from build123d import *

# Parameters (mm, degrees)
BOX013_W               = 80
BOX013_H               = 4
BOX013_DEPTH           = 80
BOX013_PLACEMENT_ANGLE = 45
FILLET059_R            = 20
BOX017_W               = 80
BOX017_H               = 4
BOX017_DEPTH           = 80
BOX017_PLACEMENT_ANGLE = 45
FILLET060_R            = 20
BOX018_W               = 100
BOX018_H               = 4
BOX018_DEPTH           = 100
BOX018_PLACEMENT_ANGLE = 45
FILLET062_R            = 60
CYLINDER039_R          = 1.6
CYLINDER039_DEPTH      = 25
CYLINDER040_R          = 1.6
CYLINDER040_DEPTH      = 25
CYLINDER041_R          = 1.6
CYLINDER041_DEPTH      = 25
CYLINDER038_R          = 1.6
CYLINDER038_DEPTH      = 25
BOX014_W               = 100
BOX014_H               = 4
BOX014_DEPTH           = 100
BOX014_PLACEMENT_ANGLE = 45
FILLET061_R            = 60
BOX012_W               = 136
BOX012_H               = 4
BOX012_DEPTH           = 200
FILLET063_R            = 30
CHAMFER017_SIZE        = 2


with BuildPart() as fillet059:
    # Box013 → Box013 (new body)
    with BuildSketch(Plane.XY):
        with Locations((40, 2)):
            Rectangle(BOX013_W, BOX013_H)
    extrude(amount=BOX013_DEPTH)


with BuildPart() as fillet059_1:
    # Box013 placement: moved
    add(fillet059.part.moved(Location((-6.57, 0, 202))).rotate(Axis((-6.57, 0, 202), (0, 1, 0)), BOX013_PLACEMENT_ANGLE))

    # Fillet059
    fillet059_edges = [fillet059_1.edges().sort_by_distance(p)[0] for p in [
        (49.998542, 2, 145.431458),
    ]]
    fillet(fillet059_edges, radius=FILLET059_R)


with BuildPart() as fillet060:
    # Box017 → Box017 (new body)
    with BuildSketch(Plane.XY):
        with Locations((40, 2)):
            Rectangle(BOX017_W, BOX017_H)
    extrude(amount=BOX017_DEPTH)


with BuildPart() as fillet060_1:
    # Box017 placement: moved
    add(fillet060.part.moved(Location((-6.57, 0, -2))).rotate(Axis((-6.57, 0, -2), (0, 1, 0)), BOX017_PLACEMENT_ANGLE))

    # Fillet060
    fillet060_edges = [fillet060_1.edges().sort_by_distance(p)[0] for p in [
        (49.998542, 2, 54.568542),
    ]]
    fillet(fillet060_edges, radius=FILLET060_R)


with BuildPart() as fillet062:
    # Box018 → Box018 (new body)
    with BuildSketch(Plane.XY):
        with Locations((50, 2)):
            Rectangle(BOX018_W, BOX018_H)
    extrude(amount=BOX018_DEPTH)


with BuildPart() as fillet062_1:
    # Box018 placement: moved
    add(fillet062.part.moved(Location((48.67, 0, 100))).rotate(Axis((48.67, 0, 100), (0, 1, 0)), BOX018_PLACEMENT_ANGLE))

    # Fillet062
    fillet062_edges = [fillet062_1.edges().sort_by_distance(p)[0] for p in [
        (48.67, 2, 100),
    ]]
    fillet(fillet062_edges, radius=FILLET062_R)


with BuildPart() as obj1:
    # Cylinder039 → Cylinder039 (new body)
    with BuildSketch(Plane(origin=(113, -20, 15), x_dir=(1, 0, 0), z_dir=(0, 1, 0))):
        Circle(CYLINDER039_R)
    extrude(amount=CYLINDER039_DEPTH)


with BuildPart() as obj2:
    # Cylinder040 → Cylinder040 (new body)
    with BuildSketch(Plane(origin=(-13, -20, 193), x_dir=(1, 0, 0), z_dir=(0, 1, 0))):
        Circle(CYLINDER040_R)
    extrude(amount=CYLINDER040_DEPTH)


with BuildPart() as obj3:
    # Cylinder041 → Cylinder041 (new body)
    with BuildSketch(Plane(origin=(113, -20, 193), x_dir=(1, 0, 0), z_dir=(0, 1, 0))):
        Circle(CYLINDER041_R)
    extrude(amount=CYLINDER041_DEPTH)


with BuildPart() as obj4:
    # Cylinder038 → Cylinder038 (new body)
    with BuildSketch(Plane(origin=(-13, -20, 15), x_dir=(1, 0, 0), z_dir=(0, 1, 0))):
        Circle(CYLINDER038_R)
    extrude(amount=CYLINDER038_DEPTH)

    # Fusion019: union obj1, obj2, obj3
    add(obj1.part)
    add(obj2.part)
    add(obj3.part)


with BuildPart() as fusion023:
    # Box014 → Box014 (new body)
    with BuildSketch(Plane.XY):
        with Locations((50, 2)):
            Rectangle(BOX014_W, BOX014_H)
    extrude(amount=BOX014_DEPTH)


with BuildPart() as fusion023_1:
    # Box014 placement: moved
    add(fusion023.part.moved(Location((-90, 0, 100))).rotate(Axis((-90, 0, 100), (0, 1, 0)), BOX014_PLACEMENT_ANGLE))

    # Fillet061
    fillet061_edges = [fusion023_1.edges().sort_by_distance(p)[0] for p in [
        (51.421356, 2, 100),
    ]]
    fillet(fillet061_edges, radius=FILLET061_R)

    # Fusion023: union Fillet059, Fillet060, Fillet062, obj4
    add(fillet059_1.part)
    add(fillet060_1.part)
    add(fillet062_1.part)
    add(obj4.part)


with BuildPart() as support:
    # Box012 → Box012 (new body)
    with BuildSketch(Plane(origin=(-18, 0, 0), x_dir=(1, 0, 0), z_dir=(0, 0, 1))):
        with Locations((68, 2)):
            Rectangle(BOX012_W, BOX012_H)
    extrude(amount=BOX012_DEPTH)

    # Cut008: cut Fusion023
    add(fusion023_1.part, mode=Mode.SUBTRACT)

    # Fillet063
    fillet063_edges = [support.edges().sort_by_distance(p)[0] for p in [
        (-18, 2, 30.578644),
        (118, 2, 30.67),
        (118, 2, 169.33),
        (-18, 2, 169.421356),
    ]]
    fillet(fillet063_edges, radius=FILLET063_R)

    # Chamfer017
    chamfer017_edges = [support.edges().sort_by_distance(p)[0] for p in [
        (-14.6, 0, 15),
        (-14.6, 0, 193),
        (111.4, 0, 15),
        (111.4, 0, 193),
    ]]
    chamfer(chamfer017_edges, length=CHAMFER017_SIZE)


solid = support.part
Can you work these out from the model? Positions are in its coordinate system, mm. A direction names the side the tool comes from. Give positions to 0.01 mm unless a question says otherwise; leave off trailing zeros. Loops run counter-clockwise (first coordinate to the right, second up) from the corner with the lowest first, then second, coordinate; pieces in that order, holes last. Notation, with made-up numbers: (-19.75, 30.25) - (35.25, 30.25) arc R16 cw to (35.25, 54.25) - close; hole circle Ø4 at (71, 10.25). An arc over 180 degrees is marked (long way). Return JSON: item names as keys, results as strings.
1. I'm going to push a flat-ended pin straight in: pin 1 Ø5 at (x, z) = (-13, 193) entering from -Y. Where does the tip first touch, or does it pass through?
Output values:
{"pin 1": "stops at y = 1.1"}
2. I want a section at B-B on y = 2.6. Please give me the cut outline in (x, z), and give its area (3 significant figures).
Output values:
{"outline": "(-18, 0) - (-4.57, 0) - (35.86, 40.43) arc R20 cw to (64.14, 40.43) - (104.57, 0) - (118, 0) - (118, 18.24) arc R30 ccw to (109.21, 39.46) - (91.1, 57.57) arc R60 cw to (91.1, 142.43) - (109.21, 160.54) arc R30 ccw to (118, 181.76) - (118, 200) - (104.57, 200) - (64.14, 159.57) arc R20 cw to (35.86, 159.57) - (-4.57, 200) - (-18, 200) - (-18, 181.85) arc R30 ccw to (-9.21, 160.63) - (8.99, 142.43) arc R60 cw to (8.99, 57.57) - (-9.21, 39.37) arc R30 ccw to (-18, 18.15) - close; hole circle Ø3.2 at (-13, 15); hole circle Ø3.2 at (-13, 193); hole circle Ø3.2 at (113, 15); hole circle Ø3.2 at (113, 193)", "area": "13,200 mm²"}
3. I want a section at C-C on z = 169. Please give me the cut outline in (x, y).
Output values:
{"outline": "(-15.11, 0) - (26.43, 0) - (26.43, 4) - (-15.11, 4) - close; (73.57, 0) - (115.15, 0) - (115.15, 4) - (73.57, 4) - close"}
4. I want a section at A-A on x = 97.5. Please give me the cut outline in (y, z), and give its area (3 significant figures).
Output values:
{"outline": "(0, 7.07) - (4, 7.07) - (4, 51.17) - (0, 51.17) - close; (0, 148.83) - (4, 148.83) - (4, 192.93) - (0, 192.93) - close", "area": "353 mm²"}
5. I want a section at D-D on x = 29. Please give me the cut outline in (y, z).
Output values:
{"outline": "(0, 33.57) - (4, 33.57) - (4, 166.43) - (0, 166.43) - close"}
6. We'd pull the mould along X, two halves only. Please class faces 4 (the face through (15.36, 2.03, 180.07)), 5 (the face through (49, 0, 99)), 6 (the face through (-18, 2, 9)): +X half, -X half, draft (parallel to the pull), parting line (faces both ways), or undercut.
Output values:
{"face 4": "undercut", "face 5": "draft", "face 6": "-X half"}
7. For faces 1 (the face through (115.65, 2.03, 170.12)), 2 (the face through (84.071, 1.972, 179.504)), 3 (the face through (-0.24, 2.03, 151.66)), which set-ups out of +Z, -Z, +X, -X, +Y, -Y let a thin tool reach every point of the face, with its end or its side?
Output values:
{"face 1": "+X, +Y, -Y", "face 2": "+Z, +Y, -Y", "face 3": "-X, +Y, -Y"}
8. If I drill on line 1 (Z direction, x = 113, y = 3.35); line 2 (X direction, y = 2.7, z = 193); line 3 (Z direction, x = -13, y = 2.85), over which ranges is the centre line in solid material (lowest first)?
Output values:
{"line 1": "z = 0 to 13.4, 16.6 to 34.83, 165.17 to 191.4, 194.6 to 200", "line 2": "x = -18 to -14.6, -11.4 to 2.43, 97.57 to 111.4, 114.6 to 118", "line 3": "z = 0 to 13.4, 16.6 to 34.74, 165.26 to 191.4, 194.6 to 200"}
